For this review, take the finished solid that the model builds, in its own axes (mm). Face numbers are marked on the shaded views. A direction names the side the tool comes from. Coordinates: 2 decimals unless noted, no trailing zeros. Write each loop counter-clockwise with the first axis right and the second up, starting at its lowest first coordinate (ties: lowest second). Pieces come first, ordered by that corner, then holes. Notation, with made-up numbers: M 82,7.5 L 117,7.5 A18 cw 117,36.5 Z; hole C 69,77 d3. An arc over 180 degrees is marked long. One line per question, with ' | ' between items.
from build123d import *

# Parameters (mm, degrees)
SKETCH_1_W          = 37
SKETCH_1_H          = 120
SKETCH_1_R          = 1.6
SKETCH_1_R_2        = 3
EXTRUDE_1_DEPTH     = 4
SKETCH_2_W          = 37
SKETCH_2_H          = 90
CUT_EXTRUDE_1_DEPTH = 3
SKETCH_3_W          = 17
SKETCH_3_H          = 15
CUT_EXTRUDE_2_DEPTH = 63.914624691
CHAMFER_1_SIZE      = 3
EXTRUDE_2_DEPTH     = 4
SKETCH_5_R          = 1.6
CUT_EXTRUDE_3_DEPTH = 78.351470574


with BuildPart() as part:
    # ｽｹｯﾁ1 → ﾎﾞｽ - 押し出し1 (new body)
    # profile 1 of 2: a face of its own
    with BuildSketch(Plane.XY):
        Rectangle(SKETCH_1_W, SKETCH_1_H)
        with Locations((13.5, -55)):
            Circle(SKETCH_1_R, mode=Mode.SUBTRACT)
        with Locations((13.5, -35)):
            Circle(SKETCH_1_R_2, mode=Mode.SUBTRACT)
        with Locations((-13.5, -55)):
            Circle(SKETCH_1_R, mode=Mode.SUBTRACT)
        with Locations((-13.5, -35)):
            Circle(SKETCH_1_R_2, mode=Mode.SUBTRACT)
        with Locations((13.5, 35)):
            Circle(SKETCH_1_R, mode=Mode.SUBTRACT)
        with Locations((13.5, 55)):
            Circle(SKETCH_1_R, mode=Mode.SUBTRACT)
        with Locations((-13.5, 35)):
            Circle(SKETCH_1_R, mode=Mode.SUBTRACT)
        with Locations((-13.5, 55)):
            Circle(SKETCH_1_R, mode=Mode.SUBTRACT)
    # profile 2 of 2: a face of its own
    with BuildSketch(Plane.XY):
        Polygon((-18.5, -25), (-18.5, -60), (18.5, -60), (18.5, 60), (-18.5, 60), (-18.5, 25), align=None)
        with Locations((-13.5, -55)):
            Circle(SKETCH_1_R, mode=Mode.SUBTRACT)
        with Locations((-13.5, -35)):
            Circle(SKETCH_1_R_2, mode=Mode.SUBTRACT)
        with Locations((13.5, -55)):
            Circle(SKETCH_1_R, mode=Mode.SUBTRACT)
        with Locations((13.5, -35)):
            Circle(SKETCH_1_R_2, mode=Mode.SUBTRACT)
        with Locations((-13.5, 35)):
            Circle(SKETCH_1_R, mode=Mode.SUBTRACT)
        with Locations((-13.5, 55)):
            Circle(SKETCH_1_R, mode=Mode.SUBTRACT)
        with Locations((13.5, 35)):
            Circle(SKETCH_1_R, mode=Mode.SUBTRACT)
        with Locations((13.5, 55)):
            Circle(SKETCH_1_R, mode=Mode.SUBTRACT)
    extrude(amount=EXTRUDE_1_DEPTH)

    # ｽｹｯﾁ2 → ｶｯﾄ - 押し出し1 (cut)
    with BuildSketch(Plane.XY.offset(4)):
        with Locations((0, -15)):
            Rectangle(SKETCH_2_W, SKETCH_2_H)
    extrude(amount=-CUT_EXTRUDE_1_DEPTH, mode=Mode.SUBTRACT)

    # ｽｹｯﾁ3 → ｶｯﾄ - 押し出し2 (cut, through all)
    with BuildSketch(Plane(origin=(0, 0, 0), x_dir=(-1, 0, 0), z_dir=(0, 0, -1))):
        with Locations((0, 45)):
            Rectangle(SKETCH_3_W, SKETCH_3_H)
    extrude(amount=-CUT_EXTRUDE_2_DEPTH, mode=Mode.SUBTRACT)

    # 面取り1
    chamfer_1_edges = [part.edges().sort_by_distance(p)[0] for p in [
        (8.5, 37.5, 2),
        (8.5, 52.5, 2),
        (-8.5, 52.5, 2),
        (-8.5, 37.5, 2),
    ]]
    chamfer(chamfer_1_edges, length=CHAMFER_1_SIZE)

    # ｽｹｯﾁ4 → ﾎﾞｽ - 押し出し2 (add, through all)
    with BuildSketch(Plane.XY.offset(4)):
        Polygon((18.5, 75), (18.5, 60), (-18.5, 60), (-8.5, 75), align=None)
    extrude(amount=-EXTRUDE_2_DEPTH)

    # ｽｹｯﾁ5 → ｶｯﾄ - 押し出し3 (cut, through all)
    with BuildSketch(Plane.XY.offset(4)):
        with Locations((14.5, 72)):
            Circle(SKETCH_5_R)
        with Locations((-7.9, 61.5)):
            Circle(SKETCH_5_R)
    extrude(amount=-CUT_EXTRUDE_3_DEPTH, mode=Mode.SUBTRACT)


solid = part.part
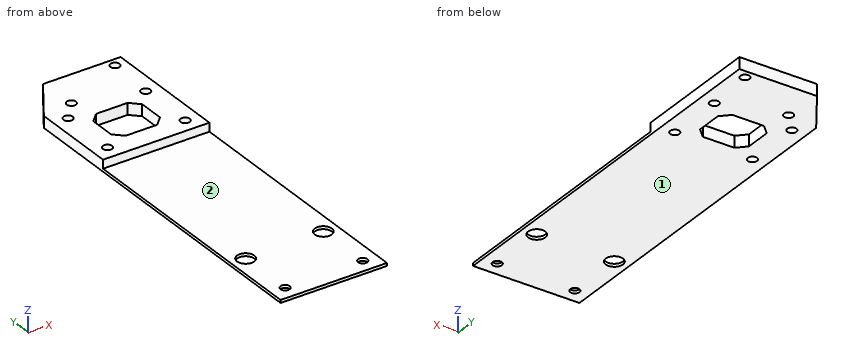
1) Machinability: for the marked faces 1 and 2, which of the approach directions +Z, -Z, +X, -X, +Y, -Y give a long, thin tool a straight path to every point of the face, cutting with its end or side? Answer none if there is none.
Responses:
face 1: -Z, +X, -X, +Y, -Y | face 2: +Z, +X, -X, -Y
2) We need section A-A on y = 72. State the section outline as (x, z) points, then the cut area to 3 significant figures.
Responses:
outline: M -10.5,0 L 12.9,0 L 12.9,4 L -10.5,4 Z; M 16.1,0 L 18.5,0 L 18.5,4 L 16.1,4 Z | area: 103 mm^2
3) We need section D-D on y = -25.5. State the section outline as (x, z) points, then the cut area to 3 significant figures.
Responses:
outline: M -18.5,0 L 18.5,0 L 18.5,1 L -18.5,1 Z | area: 37.0 mm^2
4) Insertion check: pin 1 Ø1.9 at (x, y) = (13.5, -55) entering from -Z; pin 2 Ø9.5 at (x, y) = (13.5, -35) entering from +Z. Each pin has a flat end and moves straight along its axis. Give the tip position at first contact, or say it passes through.
Responses:
pin 1: through | pin 2: z = 1
5) We need section B-B on x = -13.5. State the section outline as (y, z) points, then the cut area to 3 significant figures.
Responses:
outline: M -60,0 L -56.6,0 L -56.6,1 L -60,1 Z; M -53.4,0 L -38,0 L -38,1 L -53.4,1 Z; M -32,0 L 33.4,0 L 33.4,4 L 30,4 L 30,1 L -32,1 Z; M 36.6,0 L 53.4,0 L 53.4,4 L 36.6,4 Z; M 56.6,0 L 67.5,0 L 67.5,4 L 56.6,4 Z | area: 205 mm^2
6) To check wall thickness, follow line 1 along X through (y, z) = (-55, 0.6); line 2 along X through (y, z) = (-35, 0.7); line 3 along Y through (x, z) = (5, 1.15). State the ranges of each line that lie inside material, in increasing order. Write a range as [from, to].
Responses:
line 1: [-18.5, -15.1], [-11.9, 11.9], [15.1, 18.5] | line 2: [-18.5, -16.5], [-10.5, 10.5], [16.5, 18.5] | line 3: [30, 37.5], [52.5, 75]
7) We need section C-C on z = 2.75. State the section outline as (x, y) points, then the cut area to 3 significant figures.
Responses:
outline: M -18.5,30 L 18.5,30 L 18.5,75 L -8.5,75 L -18.5,60 Z; hole C -13.5,35 d3.2; hole C -13.5,55 d3.2; hole C -7.9,61.5 d3.2; hole M -8.5,40.5 L -5.5,37.5 L 5.5,37.5 L 8.5,40.5 L 8.5,49.5 L 5.5,52.5 L -5.5,52.5 L -8.5,49.5 Z; hole C 13.5,35 d3.2; hole C 13.5,55 d3.2; hole C 14.5,72 d3.2 | area: 1,300 mm^2
